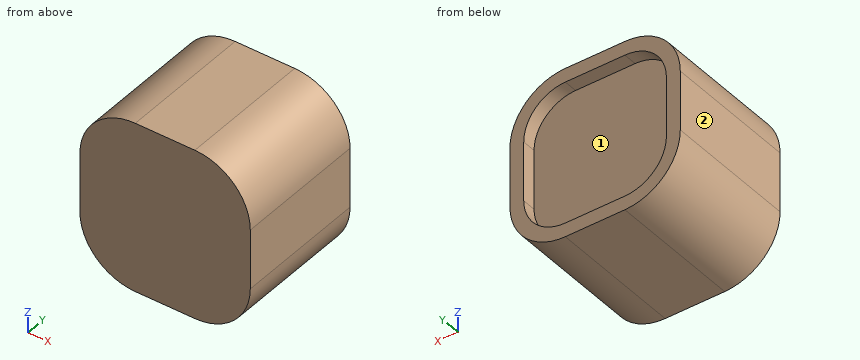
from build123d import *

# Parameters (mm, degrees)
SKETCH_1_W          = 123
SKETCH_1_H          = 123
EXTRUDE_1_DEPTH     = 97
FILLET_1_R          = 40
FILLET_2_R          = 40
FILLET_3_R          = 40
FILLET_4_R          = 40
CUT_EXTRUDE_1_DEPTH = 10


with BuildPart() as part:
    # 스케치1 → 보스-돌출1 (new body)
    with BuildSketch(Plane(origin=(0, 0, 0), x_dir=(1, 0, 0), z_dir=(0, 1, 0))):
        Rectangle(SKETCH_1_W, SKETCH_1_H)
    extrude(amount=EXTRUDE_1_DEPTH)

    # 필렛1
    fillet_1_edges = [part.edges().sort_by_distance(p)[0] for p in [
        (-61.5, 48.5, -61.5),
    ]]
    fillet(fillet_1_edges, radius=FILLET_1_R)

    # 필렛2
    fillet_2_edges = [part.edges().sort_by_distance(p)[0] for p in [
        (61.5, 48.5, -61.5),
    ]]
    fillet(fillet_2_edges, radius=FILLET_2_R)

    # 필렛3
    fillet_3_edges = [part.edges().sort_by_distance(p)[0] for p in [
        (61.5, 48.5, 61.5),
    ]]
    fillet(fillet_3_edges, radius=FILLET_3_R)

    # 필렛4
    fillet_4_edges = [part.edges().sort_by_distance(p)[0] for p in [
        (-61.5, 48.5, 61.5),
    ]]
    fillet(fillet_4_edges, radius=FILLET_4_R)

    # 스케치2 → 컷-돌출1 (cut)
    with BuildSketch(Plane(origin=(0, 97, 0), x_dir=(1, 0, 0), z_dir=(0, 1, 0))):
        with BuildLine():
            Line((21.5, 51.5), (-21.5, 51.5))
            ThreePointArc((-21.5, 51.5), (-42.713203436, 42.713203436), (-51.5, 21.5))
            Line((-51.5, 21.5), (-51.5, -21.5))
            ThreePointArc((-51.5, -21.5), (-42.713203436, -42.713203436), (-21.5, -51.5))
            Line((-21.5, -51.5), (21.5, -51.5))
            ThreePointArc((21.5, -51.5), (42.713203436, -42.713203436), (51.5, -21.5))
            Line((51.5, -21.5), (51.5, 21.5))
            ThreePointArc((51.5, 21.5), (42.713203436, 42.713203436), (21.5, 51.5))
        make_face()
    extrude(amount=-CUT_EXTRUDE_1_DEPTH, mode=Mode.SUBTRACT)


solid = part.part
Verification items for the finished model (mm, model axes). Face numbers are marked on the shaded views. A direction names the side the tool comes from. Coordinates: 2 decimals unless noted, no trailing zeros. Order: outer loops, then holes, each group sorted by start corner. A loop starts at its lowest first (then second) coordinate and runs counter-clockwise, first axis right, second up. Notation, with made-up numbers: (51, 62.5) -> (61, 62.5) arc R21 ccw to (61, 80.5) -> close; hole circle Ø9 at (6, 31). An arc over 180 degrees is marked (long way). Put each result on its own line as item: value. Start each with the question number.
1. Cross-section at B-B, the plane z = 17.5. Record the boundary of the cut face in (x, y), then the cut area to 3 significant figures.
2. Go/stop test with flat-tipped pins: pin 1 Ø1 at (y, z) = (20, -24) entering from +X; pin 2 Ø6 at (y, z) = (74.5, -38) entering from +X; pin 3 Ø3 at (y, z) = (81.5, -43) entering from +X; pin 4 Ø6 at (x, y) = (-23, 29) entering from -Z. Record where each tip stops, or that it passes through.
3. Access from +Z, -Z, +X, -X, +Y, -Y to the whole of each face (thin tool, end or side, straight path). Record for the marked faces 1 and 2.
4. Cross-section at A-A, the plane y = 63. Record the boundary of the cut face in (x, z).
5. Material ranges on L1, parallel to Y at x = 23, z = 48.5; L2, parallel to X at y = 92, z = -14; L3, parallel to X at y = 91.5, z = -35, recorded low to high. Write a range as [from, to].
Computed:
1. outline: (-61.5, 0) -> (61.5, 0) -> (61.5, 97) -> (51.5, 97) -> (51.5, 87) -> (-51.5, 87) -> (-51.5, 97) -> (-61.5, 97) -> close
1. area: 10,900 mm2
2. pin 1: x = 61.45
2. pin 2: x = 59.15
2. pin 3: x = 56.14
2. pin 4: z = -61.5
3. face 1: +Y
3. face 2: +Z, -Z, -X, +Y, -Y
4. outline: (-61.5, -21.5) arc R40 ccw to (-21.5, -61.5) -> (21.5, -61.5) arc R40 ccw to (61.5, -21.5) -> (61.5, 21.5) arc R40 ccw to (21.5, 61.5) -> (-21.5, 61.5) arc R40 ccw to (-61.5, 21.5) -> close
5. L1: [0, 87]
5. L2: [-61.5, -51.5], [51.5, 61.5]
5. L3: [-59.15, -48.29], [48.29, 59.15]
